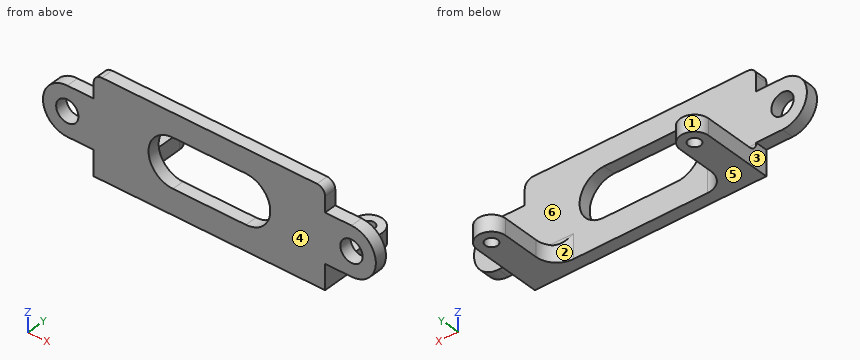
Autodesk Inventor part; units mm, degrees
ref_plane "YZ Plane" through (0, 0, 0) normal (1, 0, 0) x (0, 1, 0)
ref_plane "XZ Plane" through (0, 0, 0) normal (0, 1, 0) x (-1, 0, 0)
ref_plane "XY Plane" through (0, 0, 0) normal (0, 0, 1) x (1, 0, 0)
sketch "Sketch1" plane through (0, 0, 0) normal (0, 0, 1) x (1, 0, 0)
  line L0 (0, 0) -> (-25, 0) construction
  line L1 (0, 0) -> (25, 0) construction
  circle A0 centre (-25, 0) radius 1.5
  circle A1 centre (25, 0) radius 1.5
  line L2 (-21.5, -14) -> (21.5, -14)
  line L3 (28.5, -11.1976) -> (28.5, -17)
  line L4 (28.5, -17) -> (-28.5, -17)
  line L5 (-28.5, -17) -> (-28.5, 0.6332)
  line L6 (-21.5, -14) -> (-21.5, 0)
  line L7 (-28.5, 0) -> (-28.5, 0.6332)
  line L8 (21.5, -14) -> (21.5, 0)
  line L9 (28.5, 0) -> (28.5, -11.1976)
  arc A2 (28.5, 0) -> (21.5, 0) centre (25, 0) ccw
  arc A3 (-21.5, 0) -> (-28.5, 0) centre (-25, 0) ccw
  dimension "d0" = 50
  dimension "d1" = 3
  dimension "d2" = 3.5
  dimension "d3" = 17
  dimension "d4" = 3
extrude "Extrusion1" add sketch "Sketch1" along normal blind 4
sketch "Sketch2" plane through (0, 0, 4) normal (0, 0, 1) x (1, 0, 0)
  line L0 (28.5, -17) -> (28.5, 0)
  line L1 (28.5, -17) -> (-28.5, -17)
  line L2 (-28.5, -17) -> (-28.5, -14)
  line L3 (-28.5, -14) -> (28.5, -14)
  line L4 (28.5, -14) -> (28.5, -17)
  line L5 (-28.5, 0) -> (-28.5, -17)
  point P0 (0, 0)
  point P1 (-21.5, -14)
extrude "Extrusion2" add sketch "Sketch2" along normal blind 20
sketch "Sketch3" plane through (-28.5, -17, 0) normal (0, -1, 0) x (1, 0, 0)
  line L0 (28.5, 0) -> (28.5, 12.2) construction
  line L1 (-6.5, 12.2) -> (63.5, 12.2) construction
  line L2 (0, 24) -> (57, 24)
  line L3 (-6.5, 6.2) -> (63.5, 6.2)
  line L4 (63.5, 18.2) -> (-6.5, 18.2)
  arc A0 (-6.5, 18.2) -> (-6.5, 6.2) centre (-6.5, 12.2) ccw
  arc A1 (63.5, 6.2) -> (63.5, 18.2) centre (63.5, 12.2) ccw
  line L5 (0, 4) -> (7, 4)
  circle A2 centre (-6.5, 12.2) radius 2.75
  circle A3 centre (63.5, 12.2) radius 2.75
  dimension "d9" = 6
  dimension "d10" = 70
  dimension "d11" = 8.2
  dimension "d12" = 5.5
extrude "Extrusion3" add sketch "Sketch3" against normal up to surface (3 mm away)
sketch "Sketch4" plane through (-21.5, -14, 0) normal (0, 1, 0) x (1, 0, 0)
  circle A0 centre (-13.5, -12.2) radius 2.75 construction
  line L0 (-13.5, -12.2) -> (21.5, -12.2) construction
  line L1 (21.5, -12.2) -> (21.5, 0) construction
  line L2 (-7, 0) -> (50, 0) construction
  line L3 (30.5, -12.2) -> (12.5, -12.2) construction
  line L4 (30.5, -6.2) -> (12.5, -6.2)
  line L5 (12.5, -18.2) -> (30.5, -18.2)
  arc A1 (30.5, -18.2) -> (30.5, -6.2) centre (30.5, -12.2) ccw
  arc A2 (12.5, -6.2) -> (12.5, -18.2) centre (12.5, -12.2) ccw
  dimension "d15" = 6
  dimension "d16" = 18
extrude "Extrusion4" cut sketch "Sketch4" against normal through all
fillet "Fillet1" radius 2 2 edges at (-28.5, -15.5, 24) (28.5, -15.5, 24)
fillet "Fillet2" radius 2 2 edges at (-25, -14, 4) (25, -14, 4)
fillet "Fillet3" radius 5 4 edges at (-21.5, -14, 5) (-21.5, -14, 2) (21.5, -14, 2) (21.5, -14, 5)
properties part number "IntegzaBracket"
The model under review builds one solid part; all positions refer to its coordinate system, in mm. Face numbers are marked on the shaded views. A direction names the side the tool comes from. Give positions to 0.01 mm unless a question says otherwise; leave off trailing zeros. Order: outer loops, then holes, each group sorted by start corner. A loop starts at its lowest first (then second) coordinate and runs counter-clockwise, first axis right, second up. Notation, with made-up numbers: M -38,6 L -14,6 A27 cw -14,37 Z; hole C -21.75,-20.75 d5. An arc over 180 degrees is marked long. One line per question, with ' | ' between items. Start each with the question number.
1) Mouldability with a two-part tool opening along X and no side actions: class the marked faces 1, 2, 3 and 4 as pulls with the +X half, pulls with the -X half, needs draft (parallel to the pull), parting line crosses it, or undercut.
2) Wall thickness on L1, parallel to X at y = -1.75, z = 2.25; L2, parallel to Z at x = -35, y = -15.4; L3, parallel to Y at x = -25, z = 1.3: over which ranges is each line inside the solid? List them lowest first. Write a range as from..to.
3) Consider section C-C, the plane z = 10.75. Give the boundary of the cut face in (x, y).
4) Consider section A-A, the plane x = 25. Give the boundary of the cut face in (y, z).
5) For the marked faces 5 and 6, list the 3-axis set-ups (+Z, -Z, +X, -X, +Y, -Y) from which the entire face can be reached by the end or side of a thin tool; tool diameter is ignored.
6) Consider section B-B, the plane y = -5. Give the boundary of the cut face in (x, z), then the cut area to 3 significant figures.
7) Clearance check with flat-ended pins moving along their axes: P1, Ø5, axis at x = 35, z = 12.2, coming from the +Y side; P2, Ø2.5, axis at x = 23, y = -2.5, coming from the +Z side; P3, Ø12, axis at x = -0.5, z = 10.5, coming from the +Y side; P4, Ø0.9, axis at y = -15, z = 20, coming from the -X side. State where each tip first meets the part, or that it passes through.
8) Consider section D-D, the plane y = -10.25. Give the boundary of the cut face in (x, z), then the cut area to 3 significant figures.
Found:
1) face 1: undercut | face 2: undercut | face 3: pulls with the -X half | face 4: needs draft
2) L1: x = -28.5..-21.5, 21.5..28.5 | L2: z = 6.2..9.45, 14.95..18.2 | L3: y = -17..-1.5, 1.5..3.5
3) outline: M -40.82,-17 L -37.34,-17 L -37.34,-14 L -40.82,-14 Z; M -32.66,-17 L -14.82,-17 L -14.82,-14 L -32.66,-14 Z; M 14.82,-17 L 32.66,-17 L 32.66,-14 L 14.82,-14 Z; M 37.34,-17 L 40.82,-17 L 40.82,-14 L 37.34,-14 Z
4) outline: M -17,0 L -1.5,0 L -1.5,4 L -12,4 A2 cw -14,6 L -14,24 L -17,24 Z; M 1.5,0 L 3.5,0 L 3.5,4 L 1.5,4 Z
5) face 5: -Z, +X, -X, +Y, -Y | face 6: +Z, +Y
6) outline: M -28.5,0 L -21.5,0 L -21.5,4 L -28.5,4 Z; M 21.5,0 L 28.5,0 L 28.5,4 L 21.5,4 Z | area: 56.0 mm²
7) P1: passes through | P2: stops at z = 4 | P3: stops at y = -14 | P4: stops at x = -28.5
8) outline: M -28.5,0 L -21.34,0 L -21.34,4 L -28.5,4 Z; M 21.34,0 L 28.5,0 L 28.5,4 L 21.34,4 Z | area: 57.3 mm²
